```python
from build123d import *

# Parameters (mm, degrees)
F0_R          = 0.5
F1_DEPTH      = 10
F0_R_2        = 0.75
F2_DEPTH      = 0.5
F3_R          = 0.1
F5_DEPTH      = 25
F5_DEPTH_BACK = 25
F7_DEPTH      = 25
F7_DEPTH_BACK = 25


with BuildPart() as f1:
    # F0 (on Top) → F1 (new body)
    with BuildSketch(Plane.XY):
        Circle(F0_R)
    extrude(amount=F1_DEPTH)

    # F0 (on Top) → F2 (join)
    with BuildSketch(Plane.XY):
        Circle(F0_R_2)
        Circle(F0_R, mode=Mode.SUBTRACT)
    extrude(amount=F2_DEPTH)

    # F3
    f3_edges = [f1.edges().sort_by_distance(p)[0] for p in [
        (-0.75, 0, 0),
    ]]
    fillet(f3_edges, radius=F3_R)

    # F4 (on Right) → F5 (cut, two sides)
    with BuildSketch(Plane.YZ) as f5_sk:
        Polygon((-1.2106864015, 7.4500655755), (0, 9.998658672), (0.8667384973, 7.4500655755), (0.8667384973, 10.8232041821), (-1.2106864015, 10.8232041821), (-1.2106864015, 7.4928989634), align=None)
    extrude(amount=-F5_DEPTH, mode=Mode.SUBTRACT)
    extrude(f5_sk.sketch, amount=F5_DEPTH_BACK, mode=Mode.SUBTRACT)

    # F6 (on Front) → F7 (cut, two sides)
    with BuildSketch(Plane.XZ) as f7_sk:
        Polygon((-0.8896822692, 7.1156308986), (0, 10.0040659308), (0.8585277828, 7.1156308986), (1.0901562637, 10.4937674478), (-0.8896822692, 10.4937674478), align=None)
    extrude(amount=F7_DEPTH, mode=Mode.SUBTRACT)
    extrude(f7_sk.sketch, amount=-F7_DEPTH_BACK, mode=Mode.SUBTRACT)


solid = f1.part
```
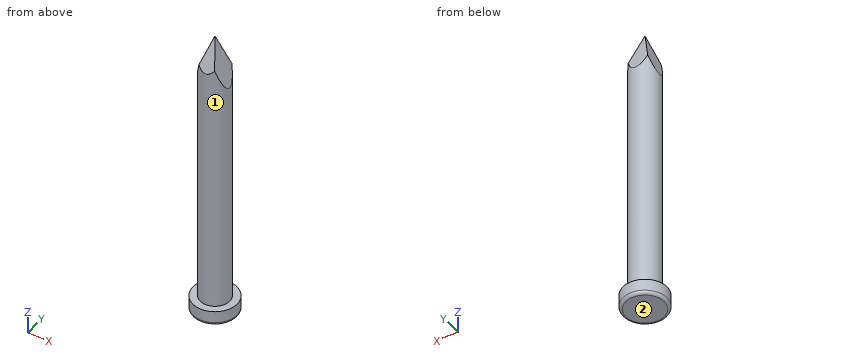
The model under review builds one solid part; all positions refer to its coordinate system, in mm. Face numbers are marked on the shaded views. A direction names the side the tool comes from. Give positions to 0.01 mm unless a question says otherwise; leave off trailing zeros. Write each loop counter-clockwise with the first axis right and the second up, starting at its lowest first coordinate (ties: lowest second). Pieces come first, ordered by that corner, then holes.
(1) Consider section A-A, the plane z = 3. Give the boundary of the cut face in (x, y).
(2) To check wall thickness, follow L1, parallel to X at y = 0.05, z = 2.75; L2, parallel to Z at x = 0.3, y = -0.45. State the ranges of each line that lie inside material, in increasing order.
(3) Tool access review of the marked faces 1 and 2: name each direction out of +Z, -Z, +X, -X, +Y, -Y from which nothing blocks a thin tool from reaching the whole face with its end or side.
Returned:
1. outline: circle Ø1 at (0, 0)
2. L1: x = -0.5 to 0.5
2. L2: z = 0 to 0.5
3. face 1: +Z
3. face 2: -Z, +X, -X, +Y, -Y
